Read the model definition and answer for the solid it produces. Units are mm, in the model's axes. A direction names the side the tool comes from. Give positions to 0.01 mm unless a question says otherwise; leave off trailing zeros. Order: outer loops, then holes, each group sorted by start corner. A loop starts at its lowest first (then second) coordinate and runs counter-clockwise, first axis right, second up. Notation, with made-up numbers: (35, 42) - (50, 42) arc R18 ccw to (50, 51) - close; hole circle Ø9 at (-30.5, -22.5). An arc over 180 degrees is marked (long way). Write item = value, one per line.
Autodesk Inventor part; units mm, degrees
ref_plane "Work Plane1" through (104.775, 0, 0) normal (0, 0, -1) x (1, 0, 0)
ref_plane "YZ Plane" through (0, 0, 0) normal (1, 0, 0) x (0, 1, 0)
ref_plane "XZ Plane" through (0, 0, 0) normal (0, 1, 0) x (-1, 0, 0)
sketch "Sketch1" plane through (0, 0, 0) normal (0, 0, 1) x (1, 0, 0)
  line L0 (30, 0) -> (30, 2)
  line L1 (30, 2) -> (10, 2)
  line L2 (10, 2) -> (9.5706, 2)
  line L3 (0, 3.765) -> (0, 1.4434)
  line L4 (0, 1.4434) -> (1.5, 1.4434)
  line L5 (1.5, 1.4434) -> (2.3333, 0)
  line L6 (2.3333, 0) -> (30, 0)
  line L7 (0, 3.765) -> (0.715, 3.765)
  line L8 (0.715, 3.765) -> (2.48, 2)
  line L9 (9.5706, 2) -> (2.48, 2)
  line L10 (10, 2) -> (2.48, 2) construction
  line L11 (2.48, 2) -> (2.48, 2)
  line L12 (-6, 0) -> (36, 0)
  line L13 (0, -0.753) -> (0, 4.518)
  dimension "d0" = 30
  dimension "d1" = 20
  dimension "d2" = 1.5
  dimension "d3" = 4
  dimension "d6" = 2.48
  dimension "d7" = 45
  dimension "d8" = 2.8868
  dimension "d9" = 60
  dimension "d10" = 7.53
  dimension "d11" = 4
  dimension "d12" = 0.4294
revolve "Body" add sketch "Sketch1" angle 360 about axis through (2.3333, 0, 0) along (1, 0, 0) contours L6 L5 L4 L3 L7 L8 L9 L2 L1 L0
sketch "Sketch2" plane through (0, 0, 0) normal (-1, 0, 0) x (0, 0, 1)
  circle A0 centre (0, 0) radius 1.4434
  line L0 (0, -5.271) -> (0, 5.271)
  line L1 (-5.271, 0) -> (5.271, 0)
  line L2 (1.4434, 0) -> (0.7217, -1.25)
  line L3 (0.7217, -1.25) -> (-0.7217, -1.25)
  line L4 (-0.7217, -1.25) -> (-1.4434, 0)
  line L5 (-1.4434, 0) -> (-0.7217, 1.25)
  line L6 (-0.7217, 1.25) -> (0.7217, 1.25)
  line L7 (0.7217, 1.25) -> (1.4434, 0)
  point P0 (0, 1.4434)
extrude "Slot" add sketch "Sketch2" against normal up to next contours L7 A0 | A0 L2 | L6 L0 A0 | A0 L0 L3 | L0 L6 A0 | A0 L3 L0 | L4 A0 | A0 L5
thread "Thread"
chamfer "Chamfer1" distance 0.4294 distance2 0.4294 1 edges at (30, -2, 0) measured on face at (30, -0.4796, 0.6016)
ref_plane "Work Plane1" through (104.775, 0, 0) normal (0, 0, -1) x (1, 0, 0)
equation "\"d15\" = GEL"
equation "\"d17\" = -0.5 * SPD + 0.5 * GD"
equation "\"d18\" = GUL"
equation "\"d0\" = NLG"
equation "\"d1\" = GEL"
equation "\"d2\" = INTI"
equation "\"d3\" = GD"
equation "\"d6\" = KOH"
equation "\"d7\" = 0.5 * SEWI"
equation "\"d8\" = 1.1547 * SW"
equation "\"d10\" = KOD"
equation "\"d11\" = BDM"
equation "\"d12\" = GAL"
equation "\"NLG\" = 30"
equation "\"INTI\" = 1.5"
equation "\"GEL\" = 20"
equation "\"GAL\" = 0.61345 * PTC"
equation "\"KOH\" = 2.48"
equation "\"KOD\" = 7.53"
equation "\"GUL\" = 0.61345 * PTC"
equation "\"SPD\" = NND - 1.2269 * PTC"
equation "\"BDM\" = NND"
equation "\"GD\" = NND"
equation "\"SEWI\" = 90deg"
equation "\"SW\" = 2.5"
equation "\"TOA\" = 30deg"
equation "\"GD1\" = THREADDIA - 1.2269 * PTC"
equation "\"EPV\" = 4.48"
equation "\"THREADDIA\" = 4"
equation "\"PTC\" = 0.7"
equation "\"NND\" = 4"
equation "\"E0\" = 1.155 * SW"
properties part number "DIN 7991 - M4  x  30" material "Steel, Mild"
1. Determine the mould class of faces 4 (the face through (30, 0, 0)), 5 (the face through (1, 1.25, 0)), 6 (the face through (0.363, -0.49, 3.733)) for opening direction Y: +Y half, -Y half, draft (parallel to the pull), parting line (faces both ways), or undercut.
Recorded:
face_4 = draft
face_5 = undercut
face_6 = parting line
2. Flat-ended cylindrical pins translate along their axes: pin 1 (2 mm diameter, centred on x = 26, y = -2.5, fed in from -Z); pin 2 (2 mm diameter, centred on x = 8.5, z = -2.5, fed in from +Y); pin 3 (1.5 mm diameter, centred on x = 20.5, y = 0, fed in from +Z). Find the tip coordinate at first contact, or state that the pin passes through.
Recorded:
pin_1 = -1.32
pin_2 = 1.32
pin_3 = 2
3. For faces 1 (the face through (16, 0, 2)), 2 (the face through (0, 0, 2)), 3 (the face through (1, -1.25, 0)), determine the directions among +Z, -Z, +X, -X, +Y, -Y from which every point of the face is accessible in a straight line to the end or side of a thin tool.
Recorded:
face_1 = +X
face_2 = +Z, -Z, -X, +Y, -Y
face_3 = -X
4. Section A-A (x = 3.5) is taken. Determine the outline of the cut face in (y, z), and give its area (3 significant figures).
Recorded:
outline = circle Ø4 at (0, 0)
area = 12.6 mm^2
5. Straight lines are drawn through the part: L1, parallel to Y at x = 18.75, z = 0.5; L2, parallel to X at y = -0.5, z = -1; L3, parallel to X at y = -1.25, z = -1.25. For each, find the intervals that lie inside material, in ascending order. Write a range as [from, to].
Recorded:
L1 = [-1.94, 1.94]
L2 = [1.69, 30]
L3 = [0, 29.8]
